Build history of the part. All positions in model axes, mm. Face numbers are marked on the shaded views. A direction names the side the tool comes from. Give positions to 0.01 mm unless a question says otherwise; leave off trailing zeros. Write each loop counter-clockwise with the first axis right and the second up, starting at its lowest first coordinate (ties: lowest second). Pieces come first, ordered by that corner, then holes. Notation, with made-up numbers: (76.5, 81.25) -> (106.5, 81.25) arc R16 cw to (106.5, 105.25) -> close; hole circle Ø5 at (76.25, 0.25). An arc over 180 degrees is marked (long way). One line per question, with ' | ' between items. Start each with the question number.
(1) Band-saw the part on B-B, the plane x = 59. Give the cut face in (y, z).
(2) Band-saw the part on A-A, the plane y = 26.5. Give the cut face in (x, z).
(3) Pin check, flat tips, straight feed: P1, Ø4, axis at x = -72.41, z = -71.76, coming from the +Y side; P2, Ø0.5, axis at y = 40, z = -72.5, coming from the -X side; P3, Ø10, axis at y = -4, z = -1.5, coming from the +X side. Stop position of each tip, or through.
(4) Tool access for the marked faces 5, 6 and 7: list every direction of +Z, -Z, +X, -X, +Y, -Y with a clear straight run to the whole face (end or side of a thin tool).
(5) Pull direction Y, two halves, no side cores. Call the marked faces 1, 2, 3 and 4: released by +Y, released by -Y, zero draft, split by the parting line, or undercut.
(6) Band-saw the part on D-D, the plane z = 0. Count the separate pieces of the cut face and the enclosed holes in it, and give its area (3 significant figures).
(7) Drill centre lines: probe 1 along X at (y, z) = (38.35, -71.76); probe 2 along Z at (x, y) = (-83.54, 39); probe 3 along Z at (x, y) = (-72, 39). Where is each one in solid material? Low to high. Write a range as from..to.
(8) Band-saw the part on C-C, the plane y = -29.5. Give the cut face in (x, z), and give its area (4 significant figures).
from build123d import *

# Parameters (mm, degrees)
BOSS_EXTRUDE1_DEPTH      = 75
BOSS_EXTRUDE1_DEPTH_BACK = 75
SKETCH2_W                = 275
SKETCH2_H                = 50.8
SKETCH4_W                = 275
SKETCH4_H                = 150
SKETCH4_W_2              = 255
SKETCH4_H_2              = 130
BOSS_EXTRUDE4_DEPTH      = 40.132
SKETCH3_R                = 15
SKETCH3_R_2              = 10
BOSS_EXTRUDE2_DEPTH      = 36
SKETCH5_W                = 19.05
SKETCH5_H                = 6.48
CUT_EXTRUDE1_DEPTH       = 0.64
M2_CLEARANCE_HOLE1_D     = 2.6
M2_CLEARANCE_HOLE1_DEPTH = 2
M2_CLEARANCE_HOLE1_TIP   = 0.781118805


with BuildPart() as part:
    # Sketch2 → Boss-Extrude1 (new, two sides: drawn at the far end of the back side and taken through both)
    with BuildSketch(Plane.XY.offset(-BOSS_EXTRUDE1_DEPTH_BACK)):
        with Locations((0, -25.4)):
            Rectangle(SKETCH2_W, SKETCH2_H)
    extrude(amount=BOSS_EXTRUDE1_DEPTH + BOSS_EXTRUDE1_DEPTH_BACK)

    # Sketch4 → Boss-Extrude4 (add)
    with BuildSketch(Plane(origin=(0, 0, 0), x_dir=(1, 0, 0), z_dir=(0, 1, 0))):
        Rectangle(SKETCH4_W, SKETCH4_H)
        Rectangle(SKETCH4_W_2, SKETCH4_H_2, mode=Mode.SUBTRACT)
    extrude(amount=BOSS_EXTRUDE4_DEPTH)

    # Sketch1 → Cut-Revolve1 (revolve, cut)
    with BuildSketch(Plane.XY, mode=Mode.PRIVATE) as cut_revolve1_sk:
        with BuildLine():
            Line((-137.5, 0), (137.5, 0))
            Line((137.5, 0), (137.5, 7.747))
            add(Edge.make_bspline(
                [(119.602, 16.764), (126.446685513, 16.474787936), (132.251729161, 15.730759902), (137.5, 12.322795174), (137.5, 7.747)],
                knots=[0, 0, 0, 0, 0.656247862, 1, 1, 1, 1], degree=3))
            Line((119.602, 16.764), (65.5, 19.05))
            Line((65.5, 19.05), (-14.564, 19.05))
            add(Edge.make_bspline(
                [(-91.78, 17.399), (-84.901336541, 18.220618135), (-60.549292723, 10.012805319), (-35.82944709, 19.05), (-14.564, 19.05)],
                knots=[0, 0, 0, 0, 0.244238151, 1, 1, 1, 1], degree=3))
            Line((-91.78, 17.399), (-137.5, 11.938))
            Line((-137.5, 11.938), (-137.5, 0))
        make_face()
    revolve(cut_revolve1_sk.sketch.rotate(Axis((-137.5, 0, 0), (1, 0, 0)), 90), axis=Axis((-137.5, 0, 0), (1, 0, 0)), mode=Mode.SUBTRACT)

    # Sketch3 → Boss-Extrude2 (add)
    with BuildSketch(Plane(origin=(137.5, 0, 0), x_dir=(0, 0, -1), z_dir=(1, 0, 0))):
        Circle(SKETCH3_R)
        Circle(SKETCH3_R_2, mode=Mode.SUBTRACT)
    boss_extrude2 = extrude(amount=BOSS_EXTRUDE2_DEPTH)

    # Mirror1: Boss-Extrude2 across plane
    add(boss_extrude2.mirror(Plane(origin=(0, 0, 0), x_dir=(0, 0, 1), z_dir=(1, 0, 0))))

    # Sketch5 → Cut-Extrude1 (cut)
    with BuildSketch(Plane(origin=(0, 40.132, 0), x_dir=(1, 0, 0), z_dir=(0, 1, 0))):
        with Locations((-77.975, 71.76)):
            Rectangle(SKETCH5_W, SKETCH5_H)
        with Locations((77.975, 71.76)):
            Rectangle(SKETCH5_W, SKETCH5_H)
    extrude(amount=-CUT_EXTRUDE1_DEPTH, mode=Mode.SUBTRACT)

    # M2 Clearance Hole1
    with Locations(Plane(origin=(0, 39.492, 0), x_dir=(1, 0, 0), z_dir=(0, 1, 0))):
        with Locations((-83.54, 71.76), (-72.41, 71.76), (72.41, 71.76), (83.54, 71.76)):
            Hole(M2_CLEARANCE_HOLE1_D / 2, depth=M2_CLEARANCE_HOLE1_DEPTH)
            with Locations((0, 0, -(M2_CLEARANCE_HOLE1_DEPTH + M2_CLEARANCE_HOLE1_TIP / 2))):  # 118° drill point
                Cone(0, M2_CLEARANCE_HOLE1_D / 2, M2_CLEARANCE_HOLE1_TIP, mode=Mode.SUBTRACT)


solid = part.part
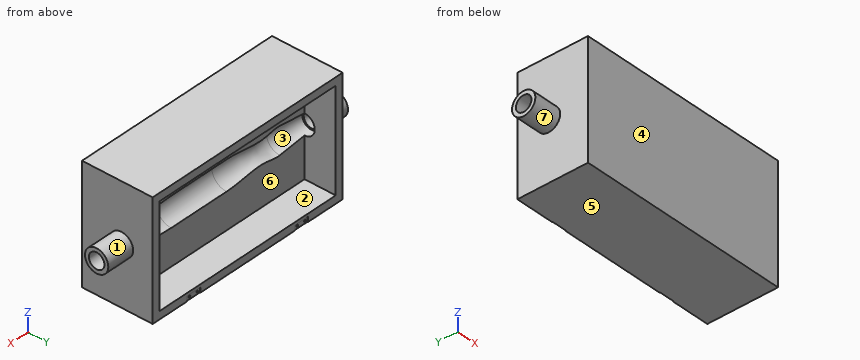
Results:
1) outline: (-50.8, -75) -> (40.13, -75) -> (40.13, -65) -> (0, -65) -> (0, -19.05) arc R19.05 cw to (0, 19.05) -> (0, 65) -> (40.13, 65) -> (40.13, 75) -> (-50.8, 75) -> close
2) outline: (-137.5, -75) -> (137.5, -75) -> (137.5, 75) -> (-137.5, 75) -> close; hole (-127.5, -65) -> (127.5, -65) -> (127.5, 65) -> (-127.5, 65) -> close
3) P1: stops at y = 39.49 | P2: stops at x = -137.5 | P3: stops at x = 137.5
4) face 5: -Z, +X, -X, +Y, -Y | face 6: +Y | face 7: -X
5) face 1: split by the parting line | face 2: zero draft | face 3: undercut | face 4: released by -Y
6) separate pieces: 3 | enclosed holes: 0 | area: 10,500 mm²
7) probe 1: x = -137.5..-84.84, -82.24..-73.71, -71.11..71.11, 73.71..82.24, 84.84..137.5 | probe 2: z = -75..-73.06, -70.46..-65, 65..75 | probe 3: z = -75..-72.99, -70.53..-65, 65..75
8) outline: (-137.5, -75) -> (137.5, -75) -> (137.5, 75) -> (-137.5, 75) -> close | area: 41,250 mm²
